CAD build for the part. Positions are in the model's coordinates, mm. A direction names the side the tool comes from. Give positions to 0.01 mm unless a question says otherwise; leave off trailing zeros. Loops run counter-clockwise (first coordinate to the right, second up) from the corner with the lowest first, then second, coordinate; pieces in that order, holes last. Notation, with made-up numbers: M 77,64.5 L 111,64.5 A21 ccw 111,95.5 Z; hole C 77.5,44.25 d8. An arc over 180 degrees is marked long. Answer as CSV lines item,"result".
```python
from build123d import *

# Parameters (mm, degrees)
BOSS_EXTRUDE1_DEPTH = 65
FILLET1_R           = 5
SKETCH2_R           = 18.75
CUT_EXTRUDE1_DEPTH  = 80
SKETCH3_R           = 23.75
CUT_EXTRUDE2_DEPTH  = 10
BOSS_EXTRUDE2_DEPTH = 65
SKETCH5_W           = 17
SKETCH5_H           = 129.632645568
CUT_EXTRUDE3_DEPTH  = 65
SKETCH6_W           = 75
SKETCH6_H           = 117.5
CUT_EXTRUDE4_DEPTH  = 60
SKETCH7_W           = 20
SKETCH7_H           = 65
BOSS_EXTRUDE3_DEPTH = 20
SKETCH8_R           = 6
CUT_EXTRUDE6_DEPTH  = 20
SKETCH9_W           = 20
SKETCH9_H           = 55
CUT_EXTRUDE8_DEPTH  = 5
SKETCH10_R          = 22.5
CUT_EXTRUDE9_DEPTH  = 7.5
SKETCH11_W          = 20
SKETCH11_H          = 10
BOSS_EXTRUDE4_DEPTH = 65
SKETCH12_R          = 5
CUT_EXTRUDE10_DEPTH = 10


with BuildPart() as part:
    # Sketch1 → Boss-Extrude1 (new body)
    with BuildSketch(Plane(origin=(0, 0, 0), x_dir=(1, 0, 0), z_dir=(0, 1, 0))):
        Polygon((0, 70), (0, -70), (-10, -80), (-155, -80), (-155, -70), (-20, -70), (-10, -60), (-10, 60), (-20, 70), (-155, 70), (-155, 80), (-10, 80), align=None)
    extrude(amount=BOSS_EXTRUDE1_DEPTH)

    # Fillet1
    fillet1_edges = [part.edges().sort_by_distance(p)[0] for p in [
        (-155, 65, 75),
        (-155, 0, -75),
        (-155, 0, 75),
        (-155, 65, -75),
    ]]
    fillet(fillet1_edges, radius=FILLET1_R)

    # Sketch2 → Cut-Extrude1 (cut)
    with BuildSketch(Plane.XY):
        with Locations((-122.5, 32.5)):
            Circle(SKETCH2_R)
    extrude(amount=-CUT_EXTRUDE1_DEPTH, mode=Mode.SUBTRACT)

    # Sketch3 → Cut-Extrude2 (cut)
    with BuildSketch(Plane.XY.offset(80)):
        with Locations((-122.5, 32.5)):
            Circle(SKETCH3_R)
    extrude(amount=-CUT_EXTRUDE2_DEPTH, mode=Mode.SUBTRACT)

    # Sketch4 → Boss-Extrude2 (add)
    with BuildSketch(Plane(origin=(0, 0, 0), x_dir=(1, 0, 0), z_dir=(0, 1, 0))):
        Polygon((-9.632645568, 79.632645568), (120, 79.632645568), (120, -70), (0, -70), (0, 70), align=None)
    extrude(amount=BOSS_EXTRUDE2_DEPTH)

    # Sketch5 → Cut-Extrude3 (cut)
    with BuildSketch(Plane.XZ):
        with Locations((6, -4.816322784)):
            Rectangle(SKETCH5_W, SKETCH5_H)
    extrude(amount=-CUT_EXTRUDE3_DEPTH, mode=Mode.SUBTRACT)

    # Sketch6 → Cut-Extrude4 (cut)
    with BuildSketch(Plane.XZ):
        with Locations((82.5, 6.25)):
            Rectangle(SKETCH6_W, SKETCH6_H)
    extrude(amount=-CUT_EXTRUDE4_DEPTH, mode=Mode.SUBTRACT)

    # Sketch7 → Boss-Extrude3 (add)
    with BuildSketch(Plane(origin=(120, 0, 0), x_dir=(0, 0, -1), z_dir=(1, 0, 0))):
        with Locations((-80, 32.5)):
            Rectangle(SKETCH7_W, SKETCH7_H)
        with Locations((89.632645568, 32.5)):
            Rectangle(SKETCH7_W, SKETCH7_H)
    extrude(amount=-BOSS_EXTRUDE3_DEPTH)

    # Sketch8 → Cut-Extrude6 (cut)
    with BuildSketch(Plane(origin=(120, 0, 0), x_dir=(0, 0, -1), z_dir=(1, 0, 0))):
        with Locations((-73.725, 32.5)):
            Circle(SKETCH8_R)
        with Locations((61.225, 32.5)):
            Circle(SKETCH8_R)
    extrude(amount=-CUT_EXTRUDE6_DEPTH, mode=Mode.SUBTRACT)

    # Sketch9 → Cut-Extrude8 (cut)
    with BuildSketch(Plane.XY.offset(70)):
        with Locations((42.5, 27.5)):
            Rectangle(SKETCH9_W, SKETCH9_H)
    extrude(amount=-CUT_EXTRUDE8_DEPTH, mode=Mode.SUBTRACT)

    # Sketch10 → Cut-Extrude9 (cut)
    with BuildSketch(Plane.ZY.offset(10)):
        with Locations((0, 30)):
            Circle(SKETCH10_R)
    extrude(amount=-CUT_EXTRUDE9_DEPTH, mode=Mode.SUBTRACT)

    # Sketch11 → Boss-Extrude4 (add)
    with BuildSketch(Plane(origin=(0, 0, 0), x_dir=(1, 0, 0), z_dir=(0, 1, 0))):
        with Locations((-85, 65)):
            Rectangle(SKETCH11_W, SKETCH11_H)
    extrude(amount=BOSS_EXTRUDE4_DEPTH)

    # Sketch12 → Cut-Extrude10 (cut)
    with BuildSketch(Plane.XY.offset(80)):
        with Locations((-68.08, 32.5)):
            Circle(SKETCH12_R)
    extrude(amount=-CUT_EXTRUDE10_DEPTH, mode=Mode.SUBTRACT)


solid = part.part
```
Q1. Wall check: line 1 (Z direction, x = -29, y = 54.5); line 2 (Y direction, x = -68, z = 76); line 3 (X direction, y = 11, z = -21). Give the ranges that are in metal, low to high. Write a range as [from, to].
Solution:
line 1,"z = [-80, -70], [70, 80]"
line 2,"y = [0, 27.5], [37.5, 65]"
line 3,"x = [-10, -2.5], [14.5, 45]"
Q2. Cut at D-D (x = -14). Write the cut outline in (y, z), and give its area (3 significant figures).
Solution:
outline,"M 0,-80 L 65,-80 L 65,-64 L 0,-64 Z; M 0,64 L 65,64 L 65,80 L 0,80 Z"
area,"2,080 mm²"
Q3. Cut at C-C (z = 45). Write the cut outline in (x, y).
Solution:
outline,"M -10,0 L -2.5,0 L -2.5,65 L -10,65 Z; M 14.5,0 L 45,0 L 45,60 L 120,60 L 120,65 L 14.5,65 Z"
Q4. Cut at A-A (x = -122.5). Write the cut outline in (y, z), and give its area (3 significant figures).
Solution:
outline,"M 0,-80 L 13.75,-80 L 13.75,-70 L 0,-70 Z; M 0,70 L 8.75,70 L 8.75,80 L 0,80 Z; M 51.25,-80 L 65,-80 L 65,-70 L 51.25,-70 Z; M 56.25,70 L 65,70 L 65,80 L 56.25,80 Z"
area,"450 mm²"
Q5. Mould opens along Y. For faces 1 (the flat face through (14.5, 32, -6)), 2 (the flat face through (100, 33, -61)) say: released by +Y, released by -Y, zero draft, split by the parting line, or undercut.
Solution:
face 1,"zero draft"
face 2,"undercut"
Q6. Pin check, flat tips, straight feed: P1, Ø8, axis at x = -79, y = 28.5, coming from the -Z side; P2, Ø4, axis at x = -50.5, z = -71.5, coming from the -Y side; P3, Ø3, axis at y = 29, z = -66.5, coming from the -X side; P4, Ø1.5, axis at x = 66, z = 41.5, coming from the -Y side. Stop position of each tip, or through.
Solution:
P1,"stops at z = -80"
P2,"stops at y = 0"
P3,"stops at x = -95"
P4,"stops at y = 60"
Q7. Which spindle directions (+Z, -Z, +X, -X, +Y, -Y) get a long thin tool onto all of the face, cutting with end or side? Do faces 3 (the flat face through (-15, 32, 65)), 4 (the flat face through (-75, 32, -65)), 5 (the flat face through (39, 28, 65)). Say none if no direction does.
Solution:
face 3,"-X, +Y, -Y"
face 4,"+Y, -Y"
face 5,"+Z, -Y"
Q8. Cut at B-B (z = 0). Write the cut outline in (x, y).
Solution:
outline,"M -10,0 L -2.5,0 L -2.5,7.5 L -10,7.5 Z; M -10,52.5 L -2.5,52.5 L -2.5,65 L -10,65 Z; M 14.5,0 L 45,0 L 45,60 L 120,60 L 120,65 L 14.5,65 Z"
